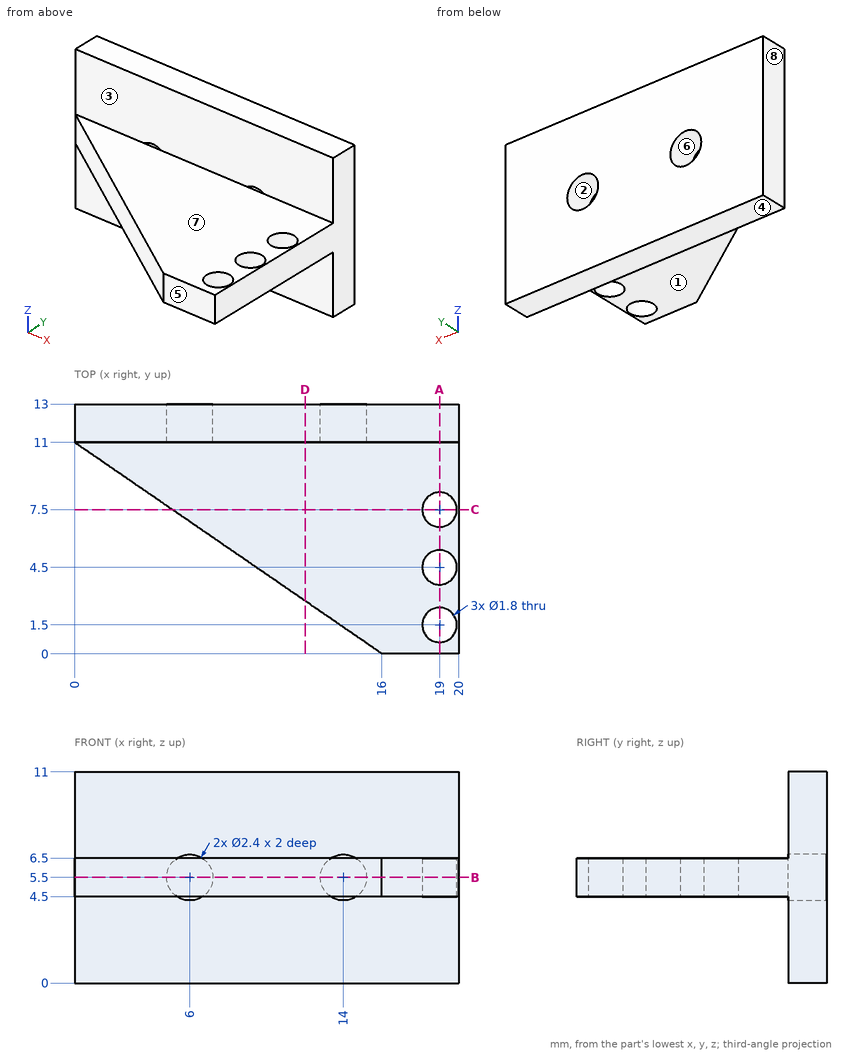
Print and shaded views of the part. All mm, measured from the part's lowest x, y and z. A direction names the side the tool comes from. Round coordinates to 2 decimals unless told otherwise and drop trailing zeros. Write each loop counter-clockwise with the first axis right and the second up, starting at its lowest first coordinate (ties: lowest second). Pieces come first, ordered by that corner, then holes. Notation, with made-up numbers: (-9, 64.25) -> (23, 64.25) arc R18 ccw to (23, 69.25) -> close; hole circle Ø11 at (-27, -35.75). An arc over 180 degrees is marked (long way). Answer in a Markdown table with one row per item. Add a question column.
Item 1: Saw through at C-C, the plane y = 7.5. Write the cut outline in (x, z), then the cut area to 3 significant figures.
Item 2: Mould opens along X. For the marked faces 6, 7 and 8 say: pulls with the +X half, pulls with the -X half, needs draft (parallel to the pull), parting line crosses it, or undercut.
Item 3: Saw through at D-D, the plane x = 12. Write the cut outline in (y, z), then the cut area to 3 significant figures.
Item 4: Saw through at A-A, the plane x = 19. Write the cut outline in (y, z), then the cut area to 3 significant figures.
Item 5: Which spindle directions (+Z, -Z, +X, -X, +Y, -Y) get a long thin tool onto all of the face, cutting with end or side? Do the marked faces 1, 2, 3, 4 and 5. Say none if no direction does.
Item 6: Saw through at B-B, the plane z = 5.5. Write the cut outline in (x, y), then the cut area to 3 significant figures.
Item 7: Drop flat-ended pins along their axis: pin 1 Ø3.5 at (x, y) = (7.5, 3) entering from +Z; pin 2 Ø1 at (x, y) = (9, 5) entering from +Z; pin 3 Ø3 at (x, z) = (3.5, 6.5) entering from -Y; pin 4 Ø1.4 at (x, z) = (14, 5.5) entering from -Y. Give the stop position or say it passes through.
Item 8: Drill centre lines: line 1 (Y direction, x = 19, z = 5.55); line 2 (X direction, y = 12.2, z = 5.5); line 3 (Z direction, x = 14, y = 11.85). Where is each one in solid material? Low to high. Write a range as from..to.
Findings below:
| question | item | result |
|---|---|---|
| 1 | outline | (5.09, 4.5) -> (18.1, 4.5) -> (18.1, 6.5) -> (5.09, 6.5) -> close; (19.9, 4.5) -> (20, 4.5) -> (20, 6.5) -> (19.9, 6.5) -> close |
| 1 | area | 26.2 mm^2 |
| 2 | face 6 | undercut |
| 2 | face 7 | needs draft |
| 2 | face 8 | pulls with the -X half |
| 3 | outline | (2.75, 4.5) -> (11, 4.5) -> (11, 0) -> (13, 0) -> (13, 11) -> (11, 11) -> (11, 6.5) -> (2.75, 6.5) -> close |
| 3 | area | 38.5 mm^2 |
| 4 | outline | (0, 4.5) -> (0.6, 4.5) -> (0.6, 6.5) -> (0, 6.5) -> close; (2.4, 4.5) -> (3.6, 4.5) -> (3.6, 6.5) -> (2.4, 6.5) -> close; (5.4, 4.5) -> (6.6, 4.5) -> (6.6, 6.5) -> (5.4, 6.5) -> close; (8.4, 4.5) -> (11, 4.5) -> (11, 0) -> (13, 0) -> (13, 11) -> (11, 11) -> (11, 6.5) -> (8.4, 6.5) -> close |
| 4 | area | 33.2 mm^2 |
| 5 | face 1 | -Z, +X, -X, -Y |
| 5 | face 2 | +Y |
| 5 | face 3 | +Z, +X, -X, -Y |
| 5 | face 4 | -Z, +X, -X, +Y, -Y |
| 5 | face 5 | +Z, -Z, +X, -X, -Y |
| 6 | outline | (0, 11) -> (16, 0) -> (20, 0) -> (20, 13) -> (15.2, 13) -> (15.2, 11) -> (12.8, 11) -> (12.8, 13) -> (7.2, 13) -> (7.2, 11) -> (4.8, 11) -> (4.8, 13) -> (0, 13) -> close; hole circle Ø1.8 at (19, 1.5); hole circle Ø1.8 at (19, 4.5); hole circle Ø1.8 at (19, 7.5) |
| 6 | area | 155 mm^2 |
| 7 | pin 1 | passes through |
| 7 | pin 2 | stops at z = 6.5 |
| 7 | pin 3 | stops at y = 7.56 |
| 7 | pin 4 | stops at y = 0.89 |
| 8 | line 1 | y = 0..0.6, 2.4..3.6, 5.4..6.6, 8.4..13 |
| 8 | line 2 | x = 0..4.8, 7.2..12.8, 15.2..20 |
| 8 | line 3 | z = 0..4.3, 6.7..11 |
